Read the model definition and answer for the solid it produces. Units are mm, in the model's axes. Face numbers are marked on the shaded views. Coordinates: 2 decimals unless noted, no trailing zeros. Loops run counter-clockwise (first coordinate to the right, second up) from the corner with the lowest first, then second, coordinate; pieces in that order, holes last.
Q1. Straight lines are drawn through the part: line 1 (Y direction, x = 0, z = 3); line 2 (Y direction, x = -2.25, z = 4.75); line 3 (X direction, y = -8, z = 2). For each, find the intervals that lie inside material, in ascending order.
Q2. The mould has two halves that part along Z. Classify the marked faces 1, 2, 3 and 4: pulls with the +Z half, pulls with the -Z half, needs draft (parallel to the pull), parting line crosses it, or undercut.
Q3. Section A-A (y = -2.25) is taken. Give the vertices of the cut face in (x, z), then the cut area to 3 significant figures.
Q4. Section B-B (z = 0) is taken. Give the vertices of the cut face in (x, y), then the cut area to 3 significant figures.
Q5. Section C-C (y = -5.5) is taken. Give the vertices of the cut face in (x, z), then the cut area to 3 significant figures.
Q6. Flat-ended cylindrical pins translate along their axes: P1, Ø2, axis at x = -3.5, y = -17.5, coming from the +Z side; P2, Ø6, axis at y = -21, z = 1.5, coming from the -X side; P3, Ø4, axis at x = -4, y = -10, coming from the -Z side; P4, Ø4, axis at x = 0, z = -5, coming from the +Y side. Find the tip coordinate at first contact, or state that the pin passes through.
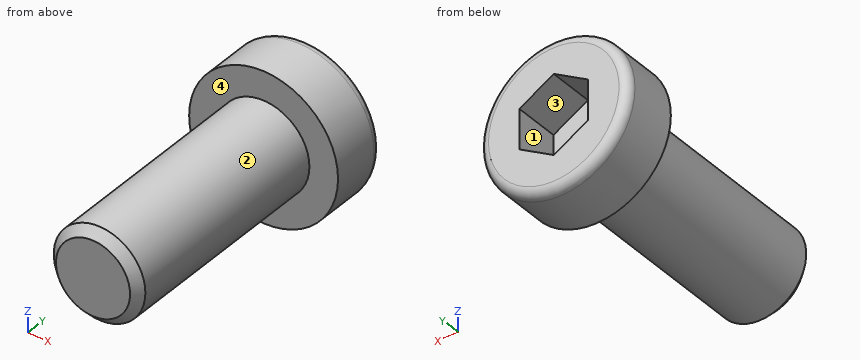
Autodesk Inventor part; units mm, degrees
ref_plane "p1_XY" through (0, -5, 0) normal (0, -1, 0) x (1, 0, 0)
ref_plane "p1_YZ" through (0, -5, 0) normal (1, 0, 0) x (0, 0, 1)
ref_plane "p1_ZX" through (0, -5, 0) normal (0, 0, 1) x (0, -1, 0)
sketch "Sketch_1" plane through (0, 0, 0) normal (0, 0, 1) x (1, 0, 0)
  line L0 (0, -50) -> (0, 50)
  line L1 (0, 0) -> (5.7, 0)
  arc A0 (6.5, -0.8) -> (5.7, 0) centre (5.7, -0.8) ccw
  line L2 (6.5, -0.8) -> (6.5, -5)
  line L3 (6.5, -5) -> (4, -5)
  line L4 (4, -5) -> (4, -24.233)
  line L5 (4, -24.233) -> (3.233, -25)
  line L6 (3.233, -25) -> (0, -25)
  line L7 (0, -25) -> (0, 0)
revolve "Revolution1" add sketch "Sketch_1" angle 360 about axis through (0, -50, 0) along (0, -1, 0)
thread "Thread1"
sketch "Sketch_2" plane through (0, 0, 0) normal (0, 1, 0) x (-1, 0, 0)
  line L0 (3, 1.7321) -> (0, 3.4641)
  line L1 (0, 3.4641) -> (-3, 1.7321)
  line L2 (-3, 1.7321) -> (-3, -1.7321)
  line L3 (-3, -1.7321) -> (0, -3.4641)
  line L4 (0, -3.4641) -> (3, -1.7321)
  line L5 (3, -1.7321) -> (3, 1.7321)
extrude "Extrusion1" cut sketch "Sketch_2" against normal blind 4
ref_plane "p1_XY" through (0, -5, 0) normal (0, -1, 0) x (1, 0, 0)
ref_plane "p1_YZ" through (0, -5, 0) normal (1, 0, 0) x (0, 0, 1)
ref_plane "p1_ZX" through (0, -5, 0) normal (0, 0, 1) x (0, -1, 0)
properties part number "Zylinderschraube DIN 6912 M8x20"
Numbers:
1. line 1: y = -25 to -4
1. line 2: y = -5 to 0
1. line 3: x = -3.46 to 3.46
2. face 1: undercut
2. face 2: parting line crosses it
2. face 3: undercut
2. face 4: needs draft
3. outline: circle Ø13 at (0, 0); hole (-3, -1.73) - (0, -3.46) - (3, -1.73) - (3, 1.73) - (0, 3.46) - (-3, 1.73) - close
3. area: 102 mm2
4. outline: (-6.5, -5) - (-4, -5) - (-4, -24.23) - (-3.23, -25) - (3.23, -25) - (4, -24.23) - (4, -5) - (6.5, -5) - (6.5, -0.8) arc R0.8 ccw to (5.7, 0) - (3, 0) - (3, -4) - (-3, -4) - (-3, 0) - (-5.7, 0) arc R0.8 ccw to (-6.5, -0.8) - close
4. area: 200 mm2
5. outline: circle Ø8 at (0, 0)
5. area: 50.3 mm2
6. P1: stops at z = 3.12
6. P2: stops at x = -4
6. P3: stops at z = -3.46
6. P4: stops at y = 0
